Verification items for the finished model (mm, model axes). A direction names the side the tool comes from. Coordinates: 2 decimals unless noted, no trailing zeros. Order: outer loops, then holes, each group sorted by start corner. A loop starts at its lowest first (then second) coordinate and runs counter-clockwise, first axis right, second up. Notation, with made-up numbers: M 49.5,52 L 107.5,52 A10 cw 107.5,64 Z; hole C 18,7.5 d3. An arc over 180 degrees is marked long. Write item = value, one per line.
```python
from build123d import *

# Parameters (mm, degrees)
SKICA2_W                 = 54.6
SKICA2_H                 = 4.2
P_IDAT_VYSUNUT_M2_DEPTH  = 0.4
SKICA3_R                 = 1.75
P_IDAT_VYSUNUT_M3_DEPTH  = 1.5
SKICA5_R                 = 1.9
P_IDAT_VYSUNUT_M5_DEPTH  = 2
ZKOSEN_2_SIZE            = 1.5
SKICA7_W                 = 1
SKICA7_H                 = 5
ODEBRAT_VYSUNUT_M1_DEPTH = 3.5


with BuildPart() as part:
    # Skica2 → Přidat vysunutím2 (new body)
    with BuildSketch(Plane.XY):
        Rectangle(SKICA2_W, SKICA2_H)
    extrude(amount=P_IDAT_VYSUNUT_M2_DEPTH)

    # Skica3 → Přidat vysunutím3 (add)
    with BuildSketch(Plane.XY.offset(0.4)):
        with Locations((-20.3, 0)):
            Circle(SKICA3_R)
        with Locations((20.3, 0)):
            Circle(SKICA3_R)
    extrude(amount=P_IDAT_VYSUNUT_M3_DEPTH)

    # Skica5 → Přidat vysunutím5 (add)
    with BuildSketch(Plane.XY.offset(1.9)):
        with Locations((-20.3, 0)):
            Circle(SKICA5_R)
        with Locations((20.3, 0)):
            Circle(SKICA5_R)
    extrude(amount=P_IDAT_VYSUNUT_M5_DEPTH)

    # Zkosení2
    zkosen_2_edges = [part.edges().sort_by_distance(p)[0] for p in [
        (-22.2, 0, 3.9),
        (18.4, 0, 3.9),
    ]]
    chamfer(zkosen_2_edges, length=ZKOSEN_2_SIZE)

    # Skica7 → Odebrat vysunutím1 (cut)
    with BuildSketch(Plane.XY.offset(3.9)):
        with Locations((-20.3, 0)):
            Rectangle(SKICA7_W, SKICA7_H)
        with Locations((20.3, 0)):
            Rectangle(SKICA7_W, SKICA7_H)
    extrude(amount=-ODEBRAT_VYSUNUT_M1_DEPTH, mode=Mode.SUBTRACT)


solid = part.part
```
Item 1: Tool access check on faces 4 (the flat face through (19.8, 0, 2)), 5 (the cylindrical face through (-18.55, -0.03, 1.14)), 6 (the cylindrical face through (-22.2, 0, 2.1)), 7 (the conical face through (-19, 0, 3)). Record the directions out of +Z, -Z, +X, -X, +Y, -Y that give a thin tool (end or side, any length) a straight path to the whole face; none if there is none.
Report:
face_4 = +Z, +Y, -Y
face_5 = none
face_6 = +Z, -X
face_7 = +Z
Item 2: Sectioned sample at A-A, the plane z = 1.05. Enter the section's corners in (x, y).
Report:
outline = M -20.8,-1.68 L -20.8,1.68 A1.75 ccw Z; M -19.8,-1.68 A1.75 ccw -19.8,1.68 Z; M 19.8,-1.68 L 19.8,1.68 A1.75 ccw Z; M 20.8,-1.68 A1.75 ccw 20.8,1.68 Z
Item 3: Release check for a two-part mould opening along Z. For faces 1 (the cylindrical face through (18.55, 0.03, 1.14)), 2 (the cylindrical face through (-18.4, 0, 2.1)), 3 (the conical face through (21.5, 0, 3.1)) record: pulls with the +Z half, pulls with the -Z half, needs draft (parallel to the pull), parting line crosses it, or undercut.
Report:
face_1 = undercut
face_2 = needs draft
face_3 = pulls with the +Z half
Item 4: Scan lines: L1, parallel to X at y = -0.1, z = 2.3; L2, parallel to X at y = -1.5, z = 2.6; L3, parallel to Z at x = 13, y = 1.55. Record each from-to range of solid material in increasing order. Write a range as from..to.
Report:
L1 = -22.2..-20.8, -19.8..-18.4, 18.4..19.8, 20.8..22.2
L2 = -21.1..-20.8, -19.8..-19.5, 19.5..19.8, 20.8..21.1
L3 = 0..0.4
Item 5: Sectioned sample at C-C, the plane x = -6. Enter the section's corners in (y, z).
Report:
outline = M -2.1,0 L 2.1,0 L 2.1,0.4 L -2.1,0.4 Z
Item 6: Gauge pin test, flat ends, axial feed: pin 1 (0.7 mm diameter, centred on x = 21.5, y = 0.5, fed in from -Z); pin 2 (1.7 mm diameter, centred on y = -0.5, z = 3, fed in from -X); pin 3 (2 mm diameter, centred on x = -12, z = 2.5, fed in from +Y); pin 4 (1.7 mm diameter, centred on y = 0, z = 1.5, fed in from +X). Record the tip position at first contact, or that the pin passes through.
Report:
pin_1 = 0
pin_2 = -22.2
pin_3 = through
pin_4 = 22.2
Item 7: Sectioned sample at B-B, the plane z = 3.25. Enter the section's corners in (x, y).
Report:
outline = M -20.8,-0.92 L -20.8,0.92 A1.05 ccw Z; M -19.8,-0.92 A1.05 ccw -19.8,0.92 Z; M 19.8,-0.92 L 19.8,0.92 A1.05 ccw Z; M 20.8,-0.92 A1.05 ccw 20.8,0.92 Z
